Check sheet for the drawn part. Datum: minimum x, y, z corner. Units: mm. A direction names the side the tool comes from. Round coordinates to 2 decimals unless told otherwise and drop trailing zeros. Write each loop counter-clockwise with the first axis right and the second up, starting at its lowest first coordinate (ties: lowest second). Pieces come first, ordered by that corner, then holes.
Item 1: Cross-section at B-B on z = 20. Enter the section's corners in (x, y).
Item 2: Cross-section at A-A on x = 19. Enter the section's corners in (y, z).
Item 3: Go/stop test with flat-tipped pins: pin 1 Ø2 at (x, z) = (22, 17.5) entering from +Y; pin 2 Ø1.5 at (x, z) = (7, 5.5) entering from -Y; pin 3 Ø3 at (y, z) = (20, 6) entering from -X; pin 4 Ø5 at (y, z) = (51.5, 11) entering from +X. Record where each tip stops, or that it passes through.
Item 4: Material ranges on line 1 (Y direction, x = 19.5, z = 17.8); line 2 (Z direction, x = 21.5, y = 19); line 3 (Y direction, x = 21.75, z = 6), recorded low to high.
Item 5: Tool access check on the marked faces 1, 2 and 3. Record the directions out of +Z, -Z, +X, -X, +Y, -Y that give a thin tool (end or side, any length) a straight path to the whole face; none if there is none.
Item 6: Cross-section at C-C on y = 52. Enter the section's corners in (x, z), plus the area to 3 significant figures.
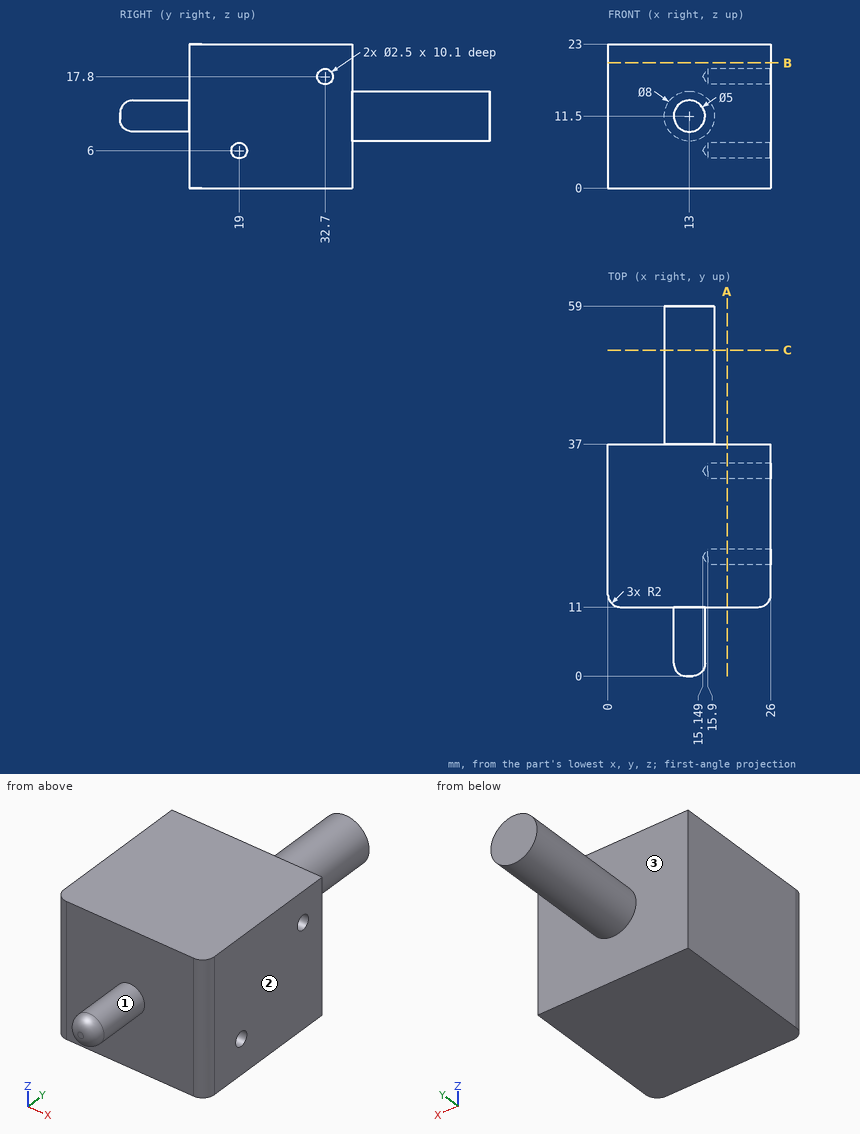
Response values:
1. outline: (0, 13) arc R2 ccw to (2, 11) - (24, 11) arc R2 ccw to (26, 13) - (26, 37) - (0, 37) - close
2. outline: (11, 0) - (37, 0) - (37, 23) - (11, 23) - close; hole circle Ø2.5 at (19, 6); hole circle Ø2.5 at (32.7, 17.8)
3. pin 1: stops at y = 37
3. pin 2: stops at y = 11
3. pin 3: stops at x = 0
3. pin 4: stops at x = 17
4. line 1: y = 11 to 31.45, 33.95 to 37
4. line 2: z = 0 to 4.75, 7.25 to 23
4. line 3: y = 11 to 17.75, 20.25 to 37
5. face 1: -Y
5. face 2: +Z, -Z, +X, +Y, -Y
5. face 3: +Y
6. outline: circle Ø8 at (13, 11.5)
6. area: 50.3 mm2
